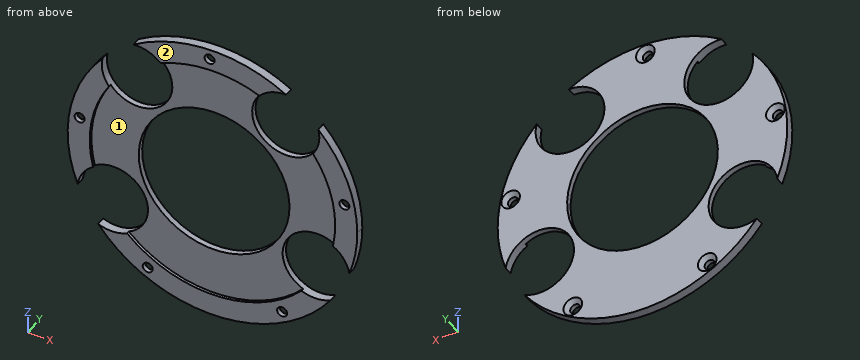
```python
from build123d import *
from build123d.topology import SkipClean

# Parameters (mm, degrees)
SKETCH1_R                                      = 25.506
BOSS_EXTRUDE1_DEPTH                            = 2
BOSS_EXTRUDE2_START                            = -3
BOSS_EXTRUDE2_DEPTH                            = 3
BOSS_EXTRUDE6_START                            = -3
BOSS_EXTRUDE6_DEPTH                            = 3
SKETCH25_R                                     = 1.7
CUT_EXTRUDE16_DEPTH                            = 95.198280418
CSK_FOR_M3_FLAT_HEAD_MACHINE_SCREW1_AT_2_COUNT = 2
CSK_FOR_M3_FLAT_HEAD_MACHINE_SCREW1_AT_2_PITCH = 45.5
CSK_FOR_M3_FLAT_HEAD_MACHINE_SCREW1_AT_3_COUNT = 2
CSK_FOR_M3_FLAT_HEAD_MACHINE_SCREW1_AT_3_PITCH = 82.47400862
CSK_FOR_M3_FLAT_HEAD_MACHINE_SCREW1_AT_4_COUNT = 2
CSK_FOR_M3_FLAT_HEAD_MACHINE_SCREW1_AT_4_PITCH = 87.899250192
CSK_FOR_M3_FLAT_HEAD_MACHINE_SCREW1_AT_5_COUNT = 2
CSK_FOR_M3_FLAT_HEAD_MACHINE_SCREW1_AT_5_PITCH = 52.195455708
CUT_EXTRUDE18_START                            = -10
SKETCH38_R                                     = 11.65
SKETCH38_R_2                                   = 10.65
CUT_EXTRUDE18_DEPTH                            = 10


with BuildPart() as part:
    # Sketch1 → Boss-Extrude1 (new body)
    with BuildSketch(Plane(origin=(0, 0, 0), x_dir=(-1, 0, 0), z_dir=(0, 1, 0))):
        with BuildLine():
            ThreePointArc((-61.273022956, -25.549853724), (-30.300207038, -39.91692623), (1.257982902, -26.885857738))
            ThreePointArc((1.257982902, -26.885857738), (-4.612463385, -11.513091013), (11.606251263, -8.731474296))
            ThreePointArc((11.606251263, -8.731474296), (12.556026093, 9.673988398), (5.631693186, 26.753705697))
            ThreePointArc((5.631693186, 26.753705697), (-10.603691781, 24.071100363), (-10.090754324, 40.518622716))
            ThreePointArc((-10.090754324, 40.518622716), (-28.482933471, 45.139662538), (-47.055700073, 41.308395969))
            ThreePointArc((-47.055700073, 41.308395969), (-47.245727944, 24.853974503), (-63.351719399, 28.227568381))
            ThreePointArc((-63.351719399, 28.227568381), (-70.999232707, 11.459185352), (-70.836448279, -6.970047687))
            ThreePointArc((-70.836448279, -6.970047687), (-54.751340848, -10.441850583), (-61.273022956, -25.549853724))
        make_face()
        with Locations(Location((-29.391570254, 2.611368154, 0), (0, 0, 90))):
            Circle(SKETCH1_R, mode=Mode.SUBTRACT)
    extrude(amount=BOSS_EXTRUDE1_DEPTH)

    # Sketch2 → Boss-Extrude2 (add)
    with SkipClean():  # the faces are left unmerged after this step: merging them gives an invalid solid
        with BuildSketch(Plane(origin=(0, 2, 0), x_dir=(1, 0, 0), z_dir=(0, 1, 0)).offset(BOSS_EXTRUDE2_START)):
            with BuildLine():
                ThreePointArc((8.100781322, -41.730874166), (9.584878111, -40.885466148), (10.914743148, -39.813683997))
                ThreePointArc((10.914743148, -39.813683997), (28.504294061, -44.139890701), (46.262572123, -40.568906798))
                ThreePointArc((46.262572123, -40.568906798), (47.545446241, -41.696511336), (48.99208013, -42.604535778))
                ThreePointArc((48.99208013, -42.604535778), (28.44021229, -47.139206211), (8.100781322, -41.730874166))
            make_face()
            with BuildLine():
                ThreePointArc((64.198332324, -30.398465127), (63.624713683, -28.789670656), (62.801291616, -27.293263594))
                ThreePointArc((62.801291616, -27.293263594), (70.021103448, -11.251187393), (69.953480433, 6.340552681))
                ThreePointArc((69.953480433, 6.340552681), (71.314539545, 7.372432563), (72.493139985, 8.608619846))
                ThreePointArc((72.493139985, 8.608619846), (72.955491227, -11.875181271), (64.198332324, -30.398465127))
            make_face()
            with BuildLine():
                ThreePointArc((63.569251617, 25.945934601), (61.87831648, 25.705110274), (60.247624932, 25.197071819))
                ThreePointArc((60.247624932, 25.197071819), (30.278846447, 38.917154393), (-0.248588426, 26.489601545))
                ThreePointArc((-0.248588426, 26.489601545), (-1.856092836, 27.066825563), (-3.535198959, 27.379652388))
                ThreePointArc((-3.535198959, 27.379652388), (30.342928218, 41.916469903), (63.569251617, 25.945934601))
            make_face()
            with BuildLine():
                ThreePointArc((-5.0418622, -25.843763068), (-5.928446542, -27.303635049), (-6.570255645, -28.886461341))
                ThreePointArc((-6.570255645, -28.886461341), (-14.528267211, -10.006050096), (-13.191445392, 10.439310852))
                ThreePointArc((-13.191445392, 10.439310852), (-12.066719813, 9.153911938), (-10.750975803, 8.064840913))
                ThreePointArc((-10.750975803, 8.064840913), (-11.569905534, -9.50795755), (-5.0418622, -25.843763068))
            make_face()
        extrude(amount=BOSS_EXTRUDE2_DEPTH)

    # Sketch24 → Boss-Extrude6 (add)
    with SkipClean():  # the faces are left unmerged after this step: merging them gives an invalid solid
        with BuildSketch(Plane(origin=(0, 2, 0), x_dir=(1, 0, 0), z_dir=(0, 1, 0)).offset(BOSS_EXTRUDE6_START)):
            with BuildLine():
                ThreePointArc((70.669999692, 23.791117773), (30.438076993, 46.377455303), (-10.721688888, 25.529819472))
                ThreePointArc((-10.721688888, 25.529819472), (-7.294770946, 27.100906435), (-3.535198959, 27.379652388))
                ThreePointArc((-3.535198959, 27.379652388), (30.342885438, 41.916470817), (63.569196745, 25.946000272))
                ThreePointArc((63.569196745, 25.946000272), (67.313347493, 25.5070047), (70.669999692, 23.791117773))
            make_face()
            with BuildLine():
                ThreePointArc((-13.191445392, 10.439310852), (-14.8672068, 13.816277617), (-15.261471823, 17.565495658))
                ThreePointArc((-15.261471823, 17.565495658), (-18.928337146, -10.746879743), (-6.19266673, -36.297597956))
                ThreePointArc((-6.19266673, -36.297597956), (-7.047830714, -32.625980412), (-6.570255645, -28.886461341))
                ThreePointArc((-6.570255645, -28.886461341), (-14.528267211, -10.006050096), (-13.191445392, 10.439310852))
            make_face()
            with BuildLine():
                ThreePointArc((78.391570254, -2.611368154), (77.502051415, 6.682802197), (74.86579056, 15.639530113))
                ThreePointArc((74.86579056, 15.639530113), (74.31165682, 11.910680729), (72.493175524, 8.608483323))
                ThreePointArc((72.493175524, 8.608483323), (72.955476555, -11.875250265), (64.198332324, -30.398465127))
                ThreePointArc((64.198332324, -30.398465127), (64.515751364, -34.154969617), (63.504547713, -37.786711349))
                ThreePointArc((63.504547713, -37.786711349), (74.516595991, -21.709327528), (78.391570254, -2.611368154))
            make_face()
            with BuildLine():
                ThreePointArc((8.100781322, -41.730874166), (4.457207722, -42.698578795), (0.704767353, -42.336263866))
                ThreePointArc((0.704767353, -42.336263866), (28.344901337, -51.600188146), (56.355487807, -43.525267384))
                ThreePointArc((56.355487807, -43.525267384), (52.590996737, -43.726979578), (48.99208013, -42.604535778))
                ThreePointArc((48.99208013, -42.604535778), (28.44021229, -47.139206211), (8.100781322, -41.730874166))
            make_face()
        extrude(amount=BOSS_EXTRUDE6_DEPTH)

    # Sketch25 → Cut-Extrude16 (cut, through all)
    with SkipClean():  # the faces are left unmerged after this step: merging them gives an invalid solid
        with BuildSketch(Plane(origin=(0.062486446, 2, -0.627225467), x_dir=(-0.9997718365651259, 0, -0.02136059014154422), z_dir=(0, 1, 0))):
            with Locations(Location((-29.391570254, 48.111368154, 0), (0, 0, 91.223964752))):
                Circle(SKETCH25_R)
            with Locations(Location((-74.200323016, 10.512360238, 0), (0, 0, 91.223964752))):
                Circle(SKETCH25_R)
            with Locations(Location((-52.141570254, -36.792787718, 0), (0, 0, 91.223964752))):
                Circle(SKETCH25_R)
            with Locations(Location((-6.641570254, -36.792787718, 0), (0, 0, 91.223964752))):
                Circle(SKETCH25_R)
            with Locations(Location((15.417182508, 10.512360238, 0), (0, 0, 91.223964752))):
                Circle(SKETCH25_R)
        extrude(amount=-CUT_EXTRUDE16_DEPTH, mode=Mode.SUBTRACT)

    # Sketch35 → CSK for M3 Flat Head Machine Screw1 (revolve, cut)
    with SkipClean():  # the faces are left unmerged after this step: merging them gives an invalid solid
        with BuildSketch(Plane(origin=(7.488456996, 2, -37.269750556), x_dir=(0, 0, 1), z_dir=(1, 0, 0))):
            Polygon((0, 0), (0, 3), (1.7, 3), (1.7, 1.45), (3.15, 0), align=None)
        csk_for_m3_flat_head_machine_screw1 = revolve(axis=Axis((7.488456996, 8.35, -37.269750556), (0, -1, 0)), mode=Mode.SUBTRACT)

    # CSK for M3 Flat Head Machine Screw1 at 2: CSK for M3 Flat Head Machine Screw1 ×2
    with SkipClean():  # the faces are left unmerged after this step: merging them gives an invalid solid
        with Locations(*[Vector(0.999771836565126, 0, 0.021360590141544296) * (i * CSK_FOR_M3_FLAT_HEAD_MACHINE_SCREW1_AT_2_PITCH) for i in range(1, CSK_FOR_M3_FLAT_HEAD_MACHINE_SCREW1_AT_2_COUNT)]):
            add(csk_for_m3_flat_head_machine_screw1, mode=Mode.SUBTRACT)

    # CSK for M3 Flat Head Machine Screw1 at 3: CSK for M3 Flat Head Machine Screw1 ×2
    with SkipClean():  # the faces are left unmerged after this step: merging them gives an invalid solid
        with Locations(*[Vector(0.8067132125731439, 0, 0.5909431382628263) * (i * CSK_FOR_M3_FLAT_HEAD_MACHINE_SCREW1_AT_3_PITCH) for i in range(1, CSK_FOR_M3_FLAT_HEAD_MACHINE_SCREW1_AT_3_COUNT)]):
            add(csk_for_m3_flat_head_machine_screw1, mode=Mode.SUBTRACT)

    # CSK for M3 Flat Head Machine Screw1 at 4: CSK for M3 Flat Head Machine Screw1 ×2
    with SkipClean():  # the faces are left unmerged after this step: merging them gives an invalid solid
        with Locations(*[Vector(0.23812724637768845, 0, 0.9712339648779689) * (i * CSK_FOR_M3_FLAT_HEAD_MACHINE_SCREW1_AT_4_PITCH) for i in range(1, CSK_FOR_M3_FLAT_HEAD_MACHINE_SCREW1_AT_4_COUNT)]):
            add(csk_for_m3_flat_head_machine_screw1, mode=Mode.SUBTRACT)

    # CSK for M3 Flat Head Machine Screw1 at 5: CSK for M3 Flat Head Machine Screw1 ×2
    with SkipClean():  # the faces are left unmerged after this step: merging them gives an invalid solid
        with Locations(*[Vector(-0.44188110488744076, 0, 0.8970736252635313) * (i * CSK_FOR_M3_FLAT_HEAD_MACHINE_SCREW1_AT_5_PITCH) for i in range(1, CSK_FOR_M3_FLAT_HEAD_MACHINE_SCREW1_AT_5_COUNT)]):
            add(csk_for_m3_flat_head_machine_screw1, mode=Mode.SUBTRACT)

    # Sketch38 → Cut-Extrude18 (cut)
    # profile 1 of 4: a face of its own
    with BuildSketch(Plane(origin=(0, 2, 0), x_dir=(1, 0, 0), z_dir=(0, 1, 0)).offset(CUT_EXTRUDE18_START)):
        with Locations((-4.639955385, 16.787107215)):
            Circle(SKETCH38_R)
        with Locations((-4.639955385, 16.787107215)):
            Circle(SKETCH38_R_2, mode=Mode.SUBTRACT)
    # profile 2 of 4: a face of its own
    with BuildSketch(Plane(origin=(0, 2, 0), x_dir=(1, 0, 0), z_dir=(0, 1, 0)).offset(CUT_EXTRUDE18_START)):
        with Locations((64.220577116, 15.315869921)):
            Circle(SKETCH38_R)
        with Locations((64.220577116, 15.315869921)):
            Circle(SKETCH38_R_2, mode=Mode.SUBTRACT)
    # profile 3 of 4: a face of its own
    with BuildSketch(Plane(origin=(0, 2, 0), x_dir=(1, 0, 0), z_dir=(0, 1, 0)).offset(CUT_EXTRUDE18_START)):
        with Locations((53.912398563, -33.159274187)):
            Circle(SKETCH38_R)
        with Locations((53.912398563, -33.159274187)):
            Circle(SKETCH38_R_2, mode=Mode.SUBTRACT)
    # profile 4 of 4: a face of its own
    with BuildSketch(Plane(origin=(0, 2, 0), x_dir=(1, 0, 0), z_dir=(0, 1, 0)).offset(CUT_EXTRUDE18_START)):
        with Locations((3.58837358, -32.084077995)):
            Circle(SKETCH38_R)
        with Locations((3.58837358, -32.084077995)):
            Circle(SKETCH38_R_2, mode=Mode.SUBTRACT)
    extrude(amount=CUT_EXTRUDE18_DEPTH, mode=Mode.SUBTRACT)


solid = part.part
```
Part model, mm, in its own coordinate system. Face numbers are marked on the shaded views. Give positions to 0.01 mm unless a question says otherwise; leave off trailing zeros. Order: outer loops, then holes, each group sorted by start corner. A loop starts at its lowest first (then second) coordinate and runs counter-clockwise, first axis right, second up. Notation, with made-up numbers: M -4,85 L 11,85 A14 ccw 11,112 Z; hole C 52.25,-31 d3. An arc over 180 degrees is marked long. Use a Markdown table: item, result. Add a question column.
(1) Saw through at B-B, the plane x = 47. Give the cut face in (y, z), and give its area (3 significant figures).
(2) Saw through at A-A, the plane x = 62. Give the cut face in (y, z), and give its area (3 significant figures).
(3) Probe line 1 along X through (y, z) = (1.75, 11.5); line 2 along X through (y, z) = (0.4, 3); line 3 along X through (y, z) = (0.5, -5). List the from-to ranges inside material, lowest first. Write a range as [from, to].
(4) Saw through at D-D, the plane z = -30.5. Give the cut face in (x, y), and give its area (3 significant figures).
(5) Saw through at C-C, the plane y = 1.4. Give the cut face in (x, z).
(6) Mould opens along Z. For the marked faces 1 and 2 say: +Z half, -Z half, draft (parallel to the pull), parting line (faces both ways), or undercut.
(7) Drop flat-ended pins along their axis: P1, Ø1.5, axis at x = 3, y = 1.5, coming from the +Z side; P2, Ø1.5, axis at x = 58.5, y = 1, coming from the +Z side; P3, Ø1.5, axis at y = 0.5, z = -10, coming from the +X side. Give the stop position or say it passes through.
Answer key:
| question | item | result |
|---|---|---|
| 1 | outline | M -1,-43.12 L 2,-43.12 L 2,-15.84 L 0,-15.84 L 0,-35.01 L -1,-35.01 Z; M -1,42.54 L 2,42.54 L 2,48.34 L -1,48.34 Z; M 0,21.06 L 2,21.06 L 2,23.78 L 0,23.78 Z |
| 1 | area | 85.5 mm^2 |
| 2 | outline | M -1,-33.96 L 2,-33.96 L 2,-26.75 L -1,-26.75 Z; M 0,-3.88 L 2,-3.88 L 2,24.77 L 0,24.77 Z |
| 2 | area | 78.9 mm^2 |
| 3 | line 1 | [-18.8, -17.73], [-13.43, 5.48], [53.3, 71.12], [76.92, 77.58] |
| 3 | line 2 | [-19.61, 3.89], [54.89, 78.39] |
| 3 | line 3 | [-19.01, 5.05], [53.74, 58.81], [69.63, 77.8] |
| 4 | outline | M -6.73,-1 L 4.31,-1 L 4.31,0 L 54.47,0 L 54.47,-1 L 65.51,-1 L 65.51,2 L -6.73,2 Z |
| 4 | area | 167 mm^2 |
| 5 | outline | M -16.2,-15.34 A11.65 cw long -9.29,-27.47 A49 ccw 69.32,-25.79 A11.65 cw long 75.71,-13.38 A49 ccw 65.19,36.07 A11.65 cw long 54.31,44.8 A49 ccw 2.69,43.7 A11.65 cw long -7.81,34.51 A49 ccw Z; hole C -15.58,9.55 d5.1; hole C 29.39,2.61 d51.01; hole C 7.49,-37.27 d5.1; hole C 28.42,48.1 d5.1; hole C 52.98,-36.3 d5.1; hole C 74.02,11.47 d5.1 |
| 6 | face 1 | undercut |
| 6 | face 2 | draft |
| 7 | P1 | z = 44.37 |
| 7 | P2 | z = 22.8 |
| 7 | P3 | x = 76.93 |
